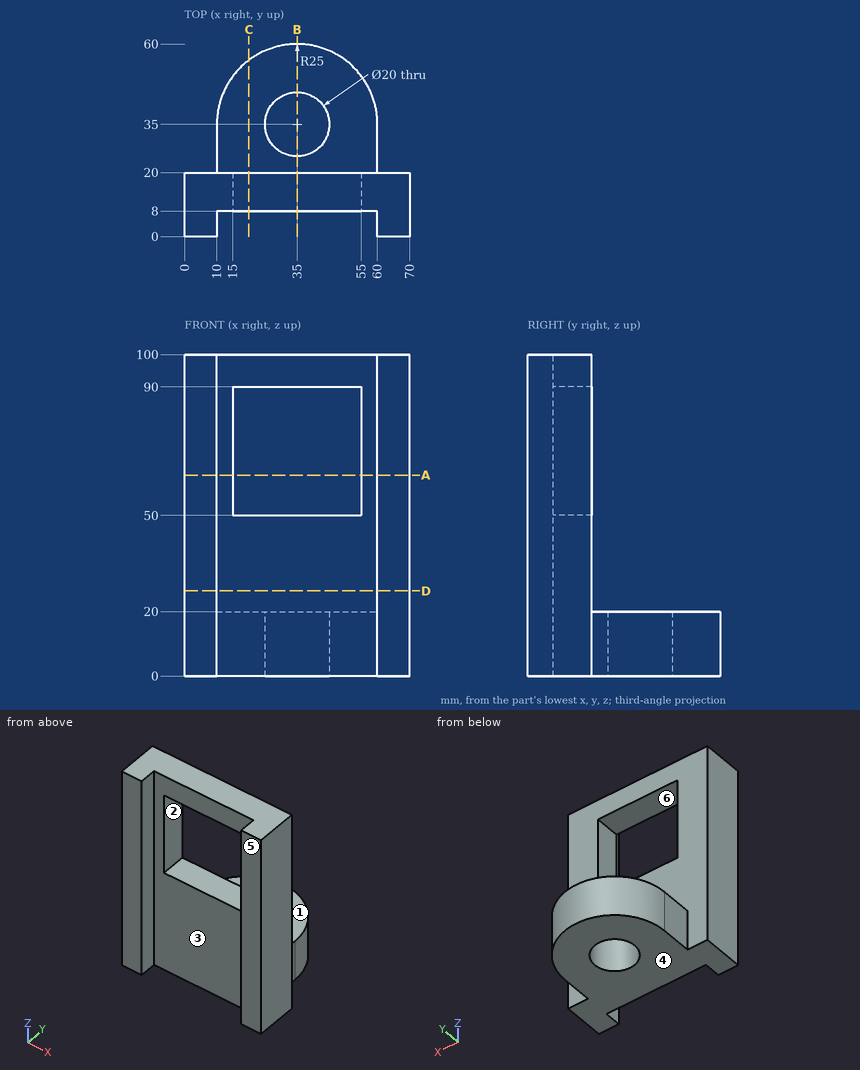
Study the drawing (mm; zero at the part's minimum x, y, z) and answer. A direction names the side the tool comes from. Round coordinates to 2 decimals unless told otherwise and drop trailing zeros. Write each loop counter-clockwise with the first axis right and the second up, starting at its lowest first coordinate (ties: lowest second). Pieces come first, ordered by that corner, then holes. Notation, with made-up numbers: (31.5, 63.5) -> (55.5, 63.5) arc R17 cw to (55.5, 81.5) -> close; hole circle Ø9 at (38, -26.75). An arc over 180 degrees is marked (long way). Use CSV: the item, a comma, the result in double quotes. Start each with the question number.
(1) Section D-D on z = 26.5 is taken. Give the vertices of the cut face in (x, y).
(2) Section C-C on x = 20 is taken. Give the vertices of the cut face in (y, z).
(3) Consider L1, parallel to Y at x = 35, z = 4.25; L2, parallel to Z at x = 40, y = 10; L3, parallel to Z at x = 53.5, y = 38. Determine where each line is inside the solid, lowest interval first. Write a range as from..to.
(4) The mould has two halves that part along Z. Classify the marked faces 4, 5 and 6: released by +Z, released by -Z, zero draft, split by the parting line, or undercut.
(5) Which of the six approach directions +Z, -Z, +X, -X, +Y, -Y give full straight-line access (tool end or side, diameter ignored) to the marked faces 1, 2 and 3?
(6) Section A-A on z = 62.5 is taken. Give the vertices of the cut face in (x, y).
(7) Each of these flat-tipped pins is pushed along its axis until it touches: pin 1 (10 mm diameter, centred on x = 55.5, z = 70.5, fed in from +Y); pin 2 (2 mm diameter, centred on x = 18, z = 47.5, fed in from -Y); pin 3 (4.5 mm diameter, centred on y = 31, z = 8, fed in from +X). Where does it stop, or does it pass through?
(8) Section B-B on x = 35 is taken. Give the vertices of the cut face in (y, z).
A:
1,outline,"(0, 0) -> (10, 0) -> (10, 8) -> (60, 8) -> (60, 0) -> (70, 0) -> (70, 20) -> (0, 20) -> close"
2,outline,"(8, 0) -> (55, 0) -> (55, 20) -> (20, 20) -> (20, 50) -> (8, 50) -> close; (8, 90) -> (20, 90) -> (20, 100) -> (8, 100) -> close"
3,L1,"y = 8..25, 45..60"
3,L2,"z = 0..50, 90..100"
3,L3,"z = 0..20"
4,face 4,"released by -Z"
4,face 5,"zero draft"
4,face 6,"undercut"
5,face 1,"+Z, +X, -X, +Y"
5,face 2,"+Y, -Y"
5,face 3,"+Z, -Z, -Y"
6,outline,"(0, 0) -> (10, 0) -> (10, 8) -> (15, 8) -> (15, 20) -> (0, 20) -> close; (55, 8) -> (60, 8) -> (60, 0) -> (70, 0) -> (70, 20) -> (55, 20) -> close"
7,pin 1,"stops at y = 20"
7,pin 2,"stops at y = 8"
7,pin 3,"stops at x = 60"
8,outline,"(8, 0) -> (25, 0) -> (25, 20) -> (20, 20) -> (20, 50) -> (8, 50) -> close; (8, 90) -> (20, 90) -> (20, 100) -> (8, 100) -> close; (45, 0) -> (60, 0) -> (60, 20) -> (45, 20) -> close"
